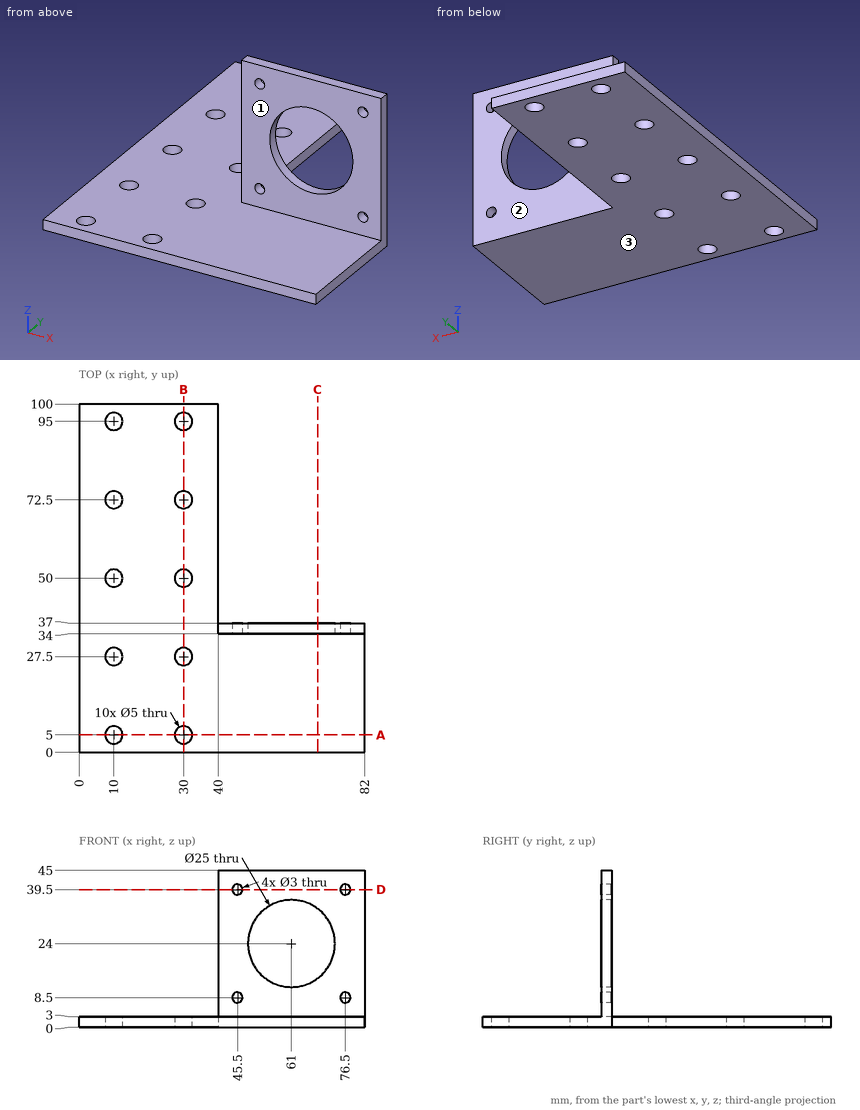
Design review of the part shown in the three views and the two pictorial views. Dimensions are in mm from the part's minimum x, y and z. A direction names the side the tool comes from. Round coordinates to 2 decimals unless told otherwise and drop trailing zeros. Loops run counter-clockwise (first coordinate to the right, second up) from the corner with the lowest first, then second, coordinate; pieces in that order, holes last. Notation, with made-up numbers: (61, 40) -> (100, 40) arc R37 ccw to (100, 77) -> close; hole circle Ø4 at (-19.75, -22.75). An arc over 180 degrees is marked (long way). Answer as a JSON object with one key per item and string values. Group by question number.
1) We need section C-C on x = 68.5. Write out the cut boundary in (y, z).
2) We need section B-B on x = 30. Write out the cut boundary in (y, z).
3) For the marked faces 1, 2 and 3, list the 3-axis set-ups (+Z, -Z, +X, -X, +Y, -Y) from which the entire face can be reached by the end or side of a thin tool; tool diameter is ignored.
4) We need section D-D on z = 39.5. Write out the cut boundary in (x, y), then the cut area to 3 significant figures.
5) For line 1 (Z direction, x = 45, y = 35); line 2 (Z direction, x = 38, y = 82); line 3 (Y direction, x = 70.5, z = 8), list the stretches that pass through material, from the lowest coordinate up. Write a range as [from, to].
6) We need section A-A on y = 5. Write out the cut boundary in (x, z), then the cut area to 3 significant figures.
7) For pin 1 Ø1 at (x, y) = (36, 21.5) entering from +Z; pin 2 Ø2.5 at (y, z) = (53.5, 1) entering from +X; pin 3 Ø3 at (x, z) = (41.5, 34) entering from -Y, all flat-tipped, find the tip position at first contact; note any pin that passes through.
Result set:
{
 "1": {"outline": "(0, 0) -> (37, 0) -> (37, 14) -> (34, 14) -> (34, 3) -> (0, 3) -> close; (34, 34) -> (37, 34) -> (37, 45) -> (34, 45) -> close"},
 "2": {"outline": "(0, 0) -> (2.5, 0) -> (2.5, 3) -> (0, 3) -> close; (7.5, 0) -> (25, 0) -> (25, 3) -> (7.5, 3) -> close; (30, 0) -> (47.5, 0) -> (47.5, 3) -> (30, 3) -> close; (52.5, 0) -> (70, 0) -> (70, 3) -> (52.5, 3) -> close; (75, 0) -> (92.5, 0) -> (92.5, 3) -> (75, 3) -> close; (97.5, 0) -> (100, 0) -> (100, 3) -> (97.5, 3) -> close"},
 "3": {"face 1": "+Z, +X, -X, -Y", "face 2": "+Z, -Z, +X, +Y", "face 3": "-Z, +X, -X, +Y, -Y"},
 "4": {"outline": "(40, 34) -> (44, 34) -> (44, 37) -> (40, 37) -> close; (47, 34) -> (75, 34) -> (75, 37) -> (47, 37) -> close; (78, 34) -> (82, 34) -> (82, 37) -> (78, 37) -> close", "area": "108 mm²"},
 "5": {"line 1": "[0, 7.09], [9.91, 38.09], [40.91, 45]", "line 2": "[0, 3]", "line 3": "[34, 37]"},
 "6": {"outline": "(0, 0) -> (7.5, 0) -> (7.5, 3) -> (0, 3) -> close; (12.5, 0) -> (27.5, 0) -> (27.5, 3) -> (12.5, 3) -> close; (32.5, 0) -> (82, 0) -> (82, 3) -> (32.5, 3) -> close", "area": "216 mm²"},
 "7": {"pin 1": "z = 3", "pin 2": "x = 40", "pin 3": "y = 34"}
}
